Can you work these out from the model? Positions are in its coordinate system, mm. Round coordinates to 2 decimals unless told otherwise and drop trailing zeros. Order: outer loops, then holes, each group sorted by start corner. A loop starts at its lowest first (then second) coordinate and runs counter-clockwise, first axis right, second up.
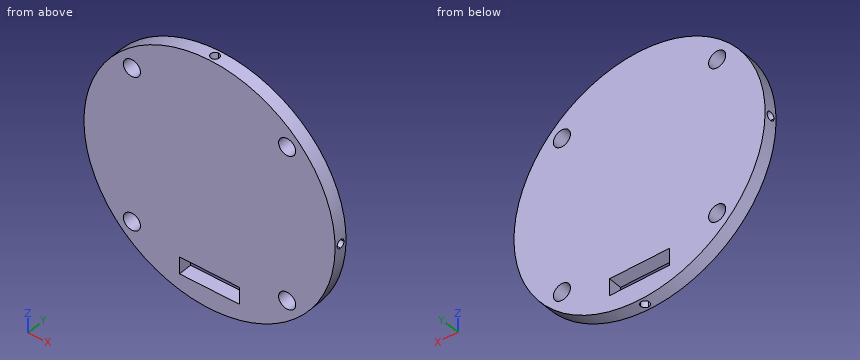
from build123d import *

# Parameters (mm, degrees)
SKETCH_1_R          = 73.5
SKETCH_1_R_2        = 5
SKETCH_1_W          = 35
SKETCH_1_H          = 10
EXTRUDE_1_DEPTH     = 8
CUT_EXTRUDE_1_DEPTH = 8
CUT_EXTRUDE_3_DEPTH = 8


with BuildPart() as part:
    # 草图1 → 凸台-拉伸1 (new body)
    with BuildSketch(Plane(origin=(0, 0, 0), x_dir=(1, 0, 0), z_dir=(0, 1, 0))):
        with Locations(Location((0, 0, 0), (0, 0, 270))):
            Circle(SKETCH_1_R)
        with Locations(Location((-45.437321384, 45.437321385, 0), (0, 0, 270))):
            Circle(SKETCH_1_R_2, mode=Mode.SUBTRACT)
        with Locations(Location((-45.437321384, -45.437321385, 0), (0, 0, 90))):
            Circle(SKETCH_1_R_2, mode=Mode.SUBTRACT)
        with Locations(Location((45.437321384, 45.437321385, 0), (0, 0, 90))):
            Circle(SKETCH_1_R_2, mode=Mode.SUBTRACT)
        with Locations(Location((45.437321384, -45.437321385, 0), (0, 0, 270))):
            Circle(SKETCH_1_R_2, mode=Mode.SUBTRACT)
        with Locations((0, 56.967179039)):
            Rectangle(SKETCH_1_W, SKETCH_1_H, mode=Mode.SUBTRACT)
    extrude(amount=EXTRUDE_1_DEPTH)

    # 草图2 → 切除-拉伸1 (cut)
    with BuildSketch(Plane.XY.offset(73.5)):
        with BuildLine():
            ThreePointArc((0, 6.5), (-2.5, 4), (0, 1.5))
            Line((0, 1.5), (0, 6.5))
        make_face()
        with BuildLine():
            Line((0, 6.5), (0, 1.5))
            ThreePointArc((0, 1.5), (1.767766953, 2.232233047), (2.5, 4))
            ThreePointArc((2.5, 4), (1.767766953, 5.767766953), (0, 6.5))
        make_face()
    cut_extrude_1 = extrude(amount=-CUT_EXTRUDE_1_DEPTH, mode=Mode.SUBTRACT)

    # 镜向1: 切除-拉伸1 across plane
    add(cut_extrude_1.mirror(Plane.XY), mode=Mode.SUBTRACT)

    # 草图3 → 切除-拉伸3 (cut)
    with BuildSketch(Plane(origin=(73.5, 0, 0), x_dir=(0, 0, -1), z_dir=(1, 0, 0))):
        with BuildLine():
            ThreePointArc((0, 6.5), (-2.5, 4), (0, 1.5))
            Line((0, 1.5), (0, 6.5))
        make_face()
        with BuildLine():
            Line((0, 6.5), (0, 1.5))
            ThreePointArc((0, 1.5), (1.767766953, 2.232233047), (2.5, 4))
            ThreePointArc((2.5, 4), (1.767766953, 5.767766953), (0, 6.5))
        make_face()
    cut_extrude_3 = extrude(amount=-CUT_EXTRUDE_3_DEPTH, mode=Mode.SUBTRACT)

    # 镜向2: 切除-拉伸3 across plane
    add(cut_extrude_3.mirror(Plane(origin=(0, 0, 0), x_dir=(0, 0, 1), z_dir=(1, 0, 0))), mode=Mode.SUBTRACT)


solid = part.part
(1) Please list where these lines run through material, in increasing order: probe 1 along Z at (x, y) = (49, 3.25); probe 2 along Z at (x, y) = (-42, 2); probe 3 along X at (y, z) = (2.25, 47).
(2) I want a section at A-A, the plane y = 5.25. List the corners of the cut face in (x, z) for me, plus the area to 3 significant figures.
(3) I want a section at D-D, the plane z = 62. List the corners of the cut face in (x, y) for me, plus the area to 3 significant figures.
(4) I want a section at B-B, the plane z = -55.5. List the corners of the cut face in (x, y) for me.
(5) I want a section at C-C, the plane x = 32. List the corners of the cut face in (y, z) for me.
(6) I'm going to push flat-ended pins straight in: pin 1 Ø1 at (x, y) = (-55.5, 4) entering from +Z; pin 2 Ø3 at (y, z) = (3, -7.5) entering from -X; pin 3 Ø2 at (y, z) = (7, 23) entering from +X; pin 4 Ø1.5 at (x, z) = (33, -13.5) entering from -Y. Where does each tip first touch, or does it pass through?
Ans:
1. probe 1: z = -54.78 to -48.95, -41.93 to 41.93, 48.95 to 54.78
1. probe 2: z = -60.32 to -49.07, -41.81 to 41.81, 49.07 to 60.32
1. probe 3: x = -56.51 to -50.19, -40.69 to 40.69, 50.19 to 56.51
2. outline: (-73.47, -2.17) arc R73.5 ccw to (-2.17, -73.47) - (-2.17, -65.5) - (2.17, -65.5) - (2.17, -73.47) arc R73.5 ccw to (73.47, -2.17) - (65.5, -2.17) - (65.5, 2.17) - (73.47, 2.17) arc R73.5 ccw to (2.17, 73.47) - (2.17, 65.5) - (-2.17, 65.5) - (-2.17, 73.47) arc R73.5 ccw to (-73.47, 2.17) - (-65.5, 2.17) - (-65.5, -2.17) - close; hole circle Ø10 at (-45.44, -45.44); hole circle Ø10 at (-45.44, 45.44); hole (-17.5, -61.97) - (17.5, -61.97) - (17.5, -51.97) - (-17.5, -51.97) - close; hole circle Ø10 at (45.44, -45.44); hole circle Ø10 at (45.44, 45.44)
2. area: 16,200 mm2
3. outline: (-39.47, 0) - (39.47, 0) - (39.47, 8) - (-39.47, 8) - close
3. area: 632 mm2
4. outline: (-48.19, 0) - (-17.5, 0) - (-17.5, 8) - (-48.19, 8) - close; (17.5, 0) - (48.19, 0) - (48.19, 8) - (17.5, 8) - close
5. outline: (0, -66.17) - (8, -66.17) - (8, 66.17) - (0, 66.17) - close
6. pin 1: stops at z = 48.76
6. pin 2: stops at x = -73.25
6. pin 3: stops at x = 70.13
6. pin 4: stops at y = 0
